Input: dimensioned drawing with shaded views. Units: mm. Origin: part minimum x, y, z. A direction names the side the tool comes from. Round coordinates to 2 decimals unless told otherwise and drop trailing zeros. Loops run counter-clockwise (first coordinate to the right, second up) from the corner with the lowest first, then second, coordinate; pieces in that order, holes last. Notation, with made-up numbers: M 30.25,-25 L 64.25,-25 A17 ccw 64.25,-8 Z; hole C 18.25,45.25 d6. An arc over 180 degrees is marked long. One line per item, written item: value.
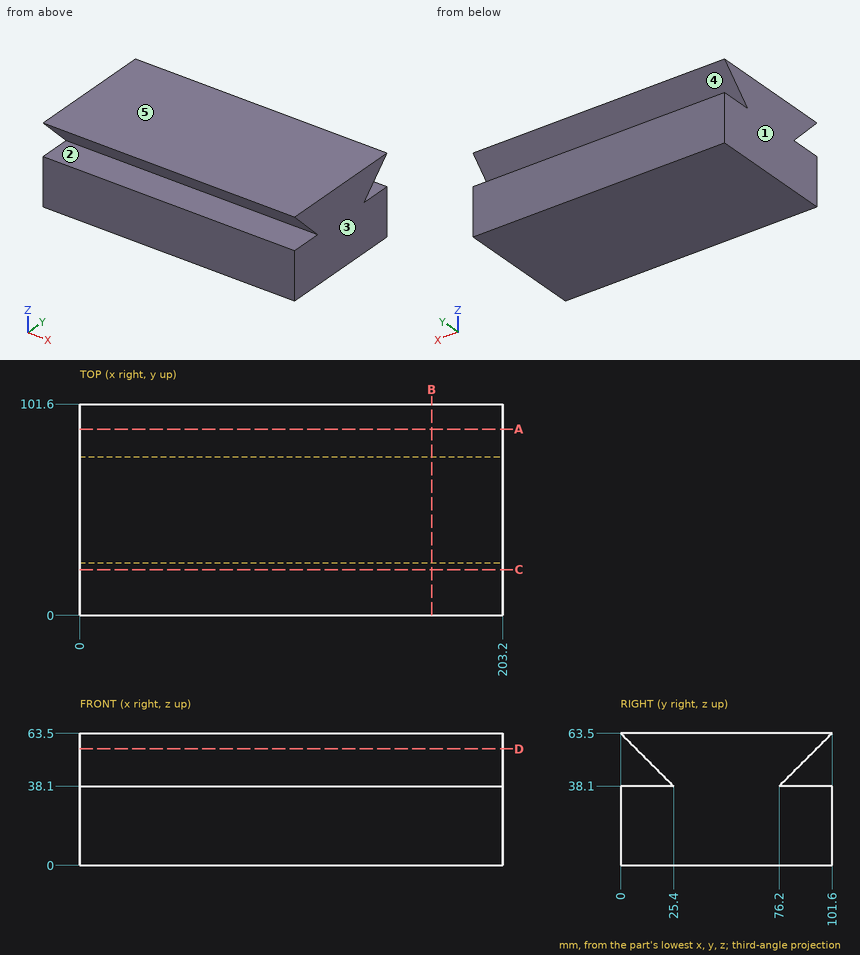
1. Section query D-D (z = 56). Return the cut outline in (x, y).
Report:
outline: M 0,7.5 L 203.2,7.5 L 203.2,94.1 L 0,94.1 Z
2. Section query A-A (y = 89.5). Return the cut outline in (x, z), and give its area (3 significant figures).
Report:
outline: M 0,0 L 203.2,0 L 203.2,38.1 L 0,38.1 Z; M 0,51.4 L 203.2,51.4 L 203.2,63.5 L 0,63.5 Z
area: 10,200 mm2
3. Reachability of the marked faces 1 and 2 from +Z, -Z, +X, -X, +Y, -Y: full face, straight path, thin tool, end or side. Return the list, or none.
Report:
face 1: +Z, -Z, -X, +Y, -Y
face 2: +X, -X, -Y
4. Pin query (flat end, axial travel): pin 1 (5 mm diameter, centred on x = 94, z = 44.5, fed in from -Y). Return the tip coordinate at first contact, or that it passes through.
Report:
pin 1: stops at y = 16.5
5. Section query B-B (x = 169). Return the cut outline in (y, z).
Report:
outline: M 0,0 L 101.6,0 L 101.6,38.1 L 76.2,38.1 L 101.6,63.5 L 0,63.5 L 25.4,38.1 L 0,38.1 Z
6. Ray query, line 1 (Z direction, x = 40.5, y = 20.5); line 2 (Z direction, x = 90, y = 79); line 3 (Y direction, x = 118.5, z = 41.5). Return the intervals inside material, ascending. Write a range as [from, to].
Report:
line 1: z = [0, 38.1], [43, 63.5]
line 2: z = [0, 38.1], [40.9, 63.5]
line 3: y = [22, 79.6]
7. Section query C-C (y = 22). Return the cut outline in (x, z).
Report:
outline: M 0,0 L 203.2,0 L 203.2,38.1 L 0,38.1 Z; M 0,41.5 L 203.2,41.5 L 203.2,63.5 L 0,63.5 Z
8. Pull-direction query (Z, two-part tool) for the marked faces 3, 4 and 5; classes: released by +Z, released by -Z, zero draft, split by the parting line, or undercut.
Report:
face 3: zero draft
face 4: undercut
face 5: released by +Z
